The listing builds one solid part. Answer for the finished solid, in the listing's coordinates (mm). A direction names the side the tool comes from. Round coordinates to 2 decimals unless told otherwise and drop trailing zeros. Order: outer loops, then holes, each group sorted by start corner. A loop starts at its lowest first (then second) coordinate and runs counter-clockwise, first axis right, second up. Notation, with made-up numbers: (43, 16) - (60, 16) arc R24 ccw to (60, 31) - close; hole circle Ø4 at (88, 73.25). An arc over 180 degrees is marked (long way). Use CSV: the item, a comma, the result in double quotes. Start each with the question number.
Item 1: Find section C-C, the plane y = 9. Give the vertices of the cut face in (x, z), plus the area to 3 significant figures.
Item 2: Find section B-B, the plane x = 37. Count the separate pieces of the cut face and the enclosed holes in it, plus the area to 3 significant figures.
Item 3: Flat-ended cylindrical pins translate along their axes: P1, Ø10, axis at x = 39.5, y = 31.5, coming from the -Z side; P2, Ø1.5, axis at x = 60.5, y = 16.5, coming from the -Z side; P3, Ø12, axis at x = 12.5, y = 61, coming from the -Z side; P4, Ø12, axis at x = 66, y = 37.5, coming from the +Z side. Find the tip coordinate at first contact, or state that the pin passes through.
Item 4: Determine the mould class of faces 1 (the flat face through (63, 0, -39)), 2 (the flat face through (46, 38, 0)), 3 (the flat face through (15.9, 38.4, -60.8)) for opening direction Y: +Y half, -Y half, draft (parallel to the pull), parting line (faces both ways), or undercut.
Item 5: For faces 4 (the flat face through (60, 69.85, -60)), 5 (the cylindrical face through (20.96, 3.69, -55.34)), 6 (the flat face through (63, 76.2, -39)), determine the directions among +Z, -Z, +X, -X, +Y, -Y from which every point of the face is accessible in a straight line to the end or side of a thin tool.
Item 6: Straight lines are drawn through the part: line 1 along Y through (x, z) = (69.5, -48.5); line 2 along Y through (x, z) = (49, -7); line 3 along X through (y, z) = (42, -60.5). For each, find the intervals that lie inside material, in ascending order. Write a range as [from, to].
Item 7: Find section A-A, the plane y = 52. Give the vertices of the cut face in (x, z), plus the area to 3 significant figures.
```python
from build123d import *

# Parameters (mm, degrees)
BOSS_EXTRUDE1_DEPTH     = 76.2
CUT_EXTRUDE4_DEPTH      = 50.546
CUT_EXTRUDE4_DEPTH_BACK = 82.042


with BuildPart() as part:
    # Sketch1 → Boss-Extrude1 (new body)
    with BuildSketch(Plane(origin=(0, 0, 0), x_dir=(1, 0, 0), z_dir=(0, 1, 0))):
        with BuildLine():
            Line((0, 0), (50.8, 0))
            ThreePointArc((50.8, 0), (68.760512242, 7.439487758), (76.2, 25.4))
            Line((76.2, 25.4), (76.2, 76.2))
            Line((76.2, 76.2), (25.4, 76.2))
            ThreePointArc((25.4, 76.2), (7.439487758, 68.760512242), (0, 50.8))
            Line((0, 50.8), (0, 0))
        make_face()
        with BuildLine():
            Line((19.05, 19.05), (50.8, 19.05))
            ThreePointArc((50.8, 19.05), (55.290128061, 20.909871939), (57.15, 25.4))
            Line((57.15, 25.4), (57.15, 57.15))
            Line((57.15, 57.15), (25.4, 57.15))
            ThreePointArc((25.4, 57.15), (20.909871939, 55.290128061), (19.05, 50.8))
            Line((19.05, 50.8), (19.05, 19.05))
        make_face(mode=Mode.SUBTRACT)
    extrude(amount=BOSS_EXTRUDE1_DEPTH)

    # Sketch3 → Cut-Extrude4 (cut, two sides)
    with BuildSketch(Plane(origin=(25.4, 0, -25.4), x_dir=(0.707106781, 0, 0.707106781), z_dir=(-0.707106781, 0, 0.707106781))) as cut_extrude4_sk:
        with BuildLine():
            Line((-31.75, 38.1), (-31.75, 19.05))
            ThreePointArc((-31.75, 19.05), (-28.030256121, 10.069743879), (-19.05, 6.35))
            Line((-19.05, 6.35), (19.05, 6.35))
            ThreePointArc((19.05, 6.35), (28.030256121, 10.069743879), (31.75, 19.05))
            Line((31.75, 19.05), (31.75, 38.1))
            Line((31.75, 38.1), (31.75, 57.15))
            ThreePointArc((31.75, 57.15), (28.030256121, 66.130256121), (19.05, 69.85))
            Line((19.05, 69.85), (-19.05, 69.85))
            ThreePointArc((-19.05, 69.85), (-28.030256121, 66.130256121), (-31.75, 57.15))
            Line((-31.75, 57.15), (-31.75, 38.1))
        make_face()
    extrude(amount=CUT_EXTRUDE4_DEPTH, mode=Mode.SUBTRACT)
    extrude(cut_extrude4_sk.sketch, amount=-CUT_EXTRUDE4_DEPTH_BACK, mode=Mode.SUBTRACT)


solid = part.part
```
Worked out:
1,outline,"(0, -50.8) arc R25.4 ccw to (25.4, -76.2) - (38.28, -76.2) - (0, -37.92) - close; (37.92, 0) - (76.2, -38.28) - (76.2, -25.4) arc R25.4 ccw to (50.8, 0) - close"
1,area,"1,190 mm²"
2,separate pieces,"4"
2,enclosed holes,"0"
2,area,"524 mm²"
3,P1,"passes through"
3,P2,"stops at z = -16.75"
3,P3,"stops at z = -75.24"
3,P4,"stops at z = -1.72"
4,face 1,"-Y half"
4,face 2,"draft"
4,face 3,"undercut"
5,face 4,"none"
5,face 5,"+Y, -Y"
5,face 6,"+Z, -Z, +X, -X, +Y"
6,line 1,"y = [0, 6.35], [69.85, 76.2]"
6,line 2,"y = [0, 12.13], [64.07, 76.2]"
6,line 3,"x = [1.93, 15.6]"
7,outline,"(0, -50.8) arc R25.4 ccw to (25.4, -76.2) - (31.3, -76.2) - (0, -44.9) - close; (44.9, 0) - (76.2, -31.3) - (76.2, -25.4) arc R25.4 ccw to (50.8, 0) - close"
7,area,"703 mm²"
